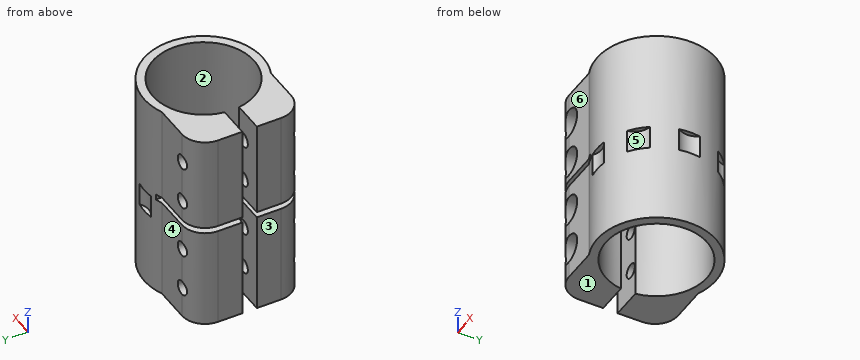
from build123d import *

# Parameters (mm, degrees)
F1_DEPTH       = 35
F3_D           = 5
F3_START       = 1.7550021
F3_CBORE_D     = 10
F3_CBORE_DEPTH = 8
F4_W           = 22.4840755326
F4_H           = 2
F5_DEPTH       = 25
F6_R           = 6
F7_DEPTH       = 8


with BuildPart() as f1:
    # F0 (on Top) → F1 (new body, symmetric)
    with BuildSketch(Plane.XY):
        with BuildLine():
            Line((-20.1192642082, -18.9086026559), (-7.9192642082, -18.9086026559))
            ThreePointArc((-7.9192642082, -18.9086026559), (20.5, 0), (-7.9192642082, 18.9086026559))
            Line((-7.9192642082, 18.9086026559), (-20.1192642082, 18.9086026559))
            ThreePointArc((-20.1192642082, 18.9086026559), (-25.7761184577, 16.5654569054), (-28.1192642082, 10.9086026559))
            Line((-28.1192642082, 10.9086026559), (-28.1192642082, 2.5086026559))
            Line((-28.1192642082, 2.5086026559), (-17.3192642082, 2.5086026559))
            ThreePointArc((-17.3192642082, 2.5086026559), (17.5, 0), (-17.3192642082, -2.5086026559))
            Line((-17.3192642082, -2.5086026559), (-28.1192642082, -2.5086026559))
            Line((-28.1192642082, -2.5086026559), (-28.1192642082, -10.9086026559))
            ThreePointArc((-28.1192642082, -10.9086026559), (-25.7761184577, -16.5654569054), (-20.1192642082, -18.9086026559))
        make_face()
    extrude(amount=F1_DEPTH, both=True)

    # F3 (through all)
    # its depths count from where the whole tool has entered the part; down to there all is cleared
    with Locations(Plane.XZ.offset(18.9086026559).offset(-F3_START)):
        with Locations((-20.1192642082, -24.25), (-20.1192642082, -9.25), (-20.1192642082, 9.25), (-20.1192642082, 24.25)):
            CounterBoreHole(F3_D / 2, F3_CBORE_D / 2, F3_CBORE_DEPTH)

    # F4 (on Front) → F5 (cut, symmetric)
    with BuildSketch(Plane.XZ):
        with Locations((-16.8772264419, 1)):
            Rectangle(F4_W, F4_H)
    extrude(amount=F5_DEPTH, both=True, mode=Mode.SUBTRACT)

    # F6 (on Top) → F7 (cut)
    with BuildSketch(Plane.XY):
        with Locations((0, -25)):
            Circle(F6_R)
        with Locations((17.6776695297, -17.6776695297)):
            Circle(F6_R)
        with Locations((25, 0)):
            Circle(F6_R)
        with Locations((17.6776695297, 17.6776695297)):
            Circle(F6_R)
        with Locations((0, 25)):
            Circle(F6_R)
    extrude(amount=-F7_DEPTH, mode=Mode.SUBTRACT)


solid = f1.part
Model file for the job. Use its own axes, mm. Face numbers are marked on the shaded views. A direction names the side the tool comes from. Give positions to 0.01 mm unless a question says otherwise; leave off trailing zeros. Order: outer loops, then holes, each group sorted by start corner. A loop starts at its lowest first (then second) coordinate and runs counter-clockwise, first axis right, second up. Notation, with made-up numbers: (27.25, 67) - (46.25, 67) arc R25 ccw to (46.25, 87) - close; hole circle Ø3 at (-10.75, -32.75). An arc over 180 degrees is marked (long way). Write item = value, one per line. Start each with the question number.
1. Two-plate mould, pull along X, no slides. Class the marked faces 1, 2 and 3: pulls with the +X half, pulls with the -X half, needs draft (parallel to the pull), parting line crosses it, or undercut.
2. Cut at B-B, the plane y = -4.5. List the corners of the cut face in (x, z), and give its area (3 significant figures).
3. Cut at A-A, the plane x = -14. List the corners of the cut face in (y, z).
4. Drop flat-ended pins along their axis: P1, Ø8, axis at y = 7, z = 7, coming from the +X side; P2, Ø3, axis at x = -18.5, z = -8.5, coming from the -Y side; P3, Ø5, axis at y = 11, z = 13.5, coming from the +X side. Give the stop position or say it passes through.
5. Cut at D-D, the plane z = -24.25. List the corners of the cut face in (x, y), and give its area (3 significant figures).
6. Which spindle directions (+Z, -Z, +X, -X, +Y, -Y) get a long thin tool onto all of the face, cutting with end or side? Do the marked faces 4, 5 and 6. Say none if no direction does.
7. Cut at C-C, the plane x = 0. List the corners of the cut face in (y, z), and give its area (3 significant figures).
8. Probe line 1 along X through (y, z) = (-5.5, -8.5); line 2 along Z through (x, y) = (-13, 13); line 3 along X through (y, z) = (-15.5, 8.5). List the from-to ranges inside material, lowest first.
Taken from the geometry:
q1.face_1 = needs draft
q1.face_2 = undercut
q1.face_3 = pulls with the -X half
q2.outline = (-28.12, -35) - (-16.91, -35) - (-16.91, 0) - (-28.12, 0) - close; (-28.12, 2) - (-16.91, 2) - (-16.91, 35) - (-28.12, 35) - close; (16.91, -35) - (20, -35) - (20, 35) - (16.91, 35) - close; hole circle Ø5 at (-20.12, -24.25); hole circle Ø5 at (-20.12, -9.25); hole circle Ø5 at (-20.12, 9.25); hole circle Ø5 at (-20.12, 24.25)
q2.area = 900 mm²
q3.outline = (-18.91, -35) - (-10.5, -35) - (-10.5, 0) - (-18.91, 0) - close; (-18.91, 2) - (-10.5, 2) - (-10.5, 35) - (-18.91, 35) - close; (10.5, -35) - (18.91, -35) - (18.91, 0) - (10.5, 0) - close; (10.5, 2) - (18.91, 2) - (18.91, 35) - (10.5, 35) - close
q4.P1 = 20.28
q4.P2 = -9.15
q4.P3 = 18.65
q5.outline = (-28.12, -10.91) arc R8 ccw to (-25.12, -17.15) - (-25.12, -9.15) - (-22.62, -9.15) - (-22.62, -2.51) - (-28.12, -2.51) - close; (-28.12, 2.51) - (-22.62, 2.51) - (-22.62, 18.51) arc R8 ccw to (-28.12, 10.91) - close; (-17.62, -9.15) - (-15.12, -9.15) - (-15.12, -18.91) - (-7.92, -18.91) arc R20.5 ccw (long way) to (-7.92, 18.91) - (-17.62, 18.91) - (-17.62, 2.51) - (-17.32, 2.51) arc R17.5 cw (long way) to (-17.32, -2.51) - (-17.62, -2.51) - close
q5.area = 488 mm²
q6.face_4 = +Z, -Z, -X, +Y
q6.face_5 = +X, -Y
q6.face_6 = +Z, -Z, -X, -Y
q7.outline = (-20.5, -35) - (-17.5, -35) - (-17.5, 35) - (-20.5, 35) - (-20.5, 0) - (-19, 0) - (-19, -8) - (-20.5, -8) - close; (17.5, -35) - (20.5, -35) - (20.5, -8) - (19, -8) - (19, 0) - (20.5, 0) - (20.5, 35) - (17.5, 35) - close
q7.area = 396 mm²
q8.line_1 = -28.12 to -22.5, -17.73 to -16.61, 16.61 to 19.75
q8.line_2 = -35 to 0, 2 to 35
q8.line_3 = -26.67 to -25.06, -15.18 to -8.12, 8.12 to 13.42
